```python
from build123d import *

# Parameters (mm, degrees)
PAD_DEPTH          = 5
POCKET_DEPTH       = 5.001
SKETCH002_R        = 5
POCKET001_DEPTH    = 5
SKETCH003_R        = 2.5
PAD001_DEPTH       = 15
POLARPATTERN_COUNT = 3


with BuildPart() as part:
    # Sketch → Pad (new body)
    with BuildSketch(Plane.XY):
        Polygon((0, 31.754265), (-27.5, -15.877132), (27.5, -15.877132), align=None)
    extrude(amount=PAD_DEPTH)

    # Sketch001 (on Face5 of Pad) → Pocket (cut, through all)
    with BuildSketch(Plane.XY.offset(5)):
        Polygon((-21.25, -5.051815), (-15, -15.877132), (-27.5, -15.877132), align=None)
        Polygon((27.5, -15.877132), (21.25, -5.051815), (15, -15.877132), align=None)
        Polygon((0, 31.754265), (6.25, 20.928947), (-6.25, 20.928947), align=None)
    extrude(amount=-POCKET_DEPTH, mode=Mode.SUBTRACT)

    # Sketch002 (on Face4 of Pocket) → Pocket001 (cut)
    with BuildSketch(Plane.XY.offset(5)):
        Circle(SKETCH002_R)
    extrude(amount=-POCKET001_DEPTH, mode=Mode.SUBTRACT)

    # Sketch003 → Pad001 (join, symmetric)
    with BuildSketch(Plane.YZ):
        with BuildLine():
            ThreePointArc((-16.02939, 13.038792), (-23.453338, 13.615862), (-23.218057, 6.173238))
            Line((-15.877132, 0), (-23.218057, 6.173238))
            Line((-15.877132, 5), (-15.877132, 0))
            Line((-9.877132, 5), (-15.877132, 5))
            Line((-16.02939, 13.038792), (-9.877132, 5))
        make_face()
        with Locations((-20, 10)):
            Circle(SKETCH003_R, mode=Mode.SUBTRACT)
    pad001 = extrude(amount=PAD001_DEPTH, both=True)

    # PolarPattern: Pad001 ×3 about axis
    polarpattern_axis = Axis((0, 0, 0), (0, 0, 1))
    for i in range(1, POLARPATTERN_COUNT):
        add(pad001.rotate(polarpattern_axis, i * 360 / POLARPATTERN_COUNT))


solid = part.part
```
Work out the finished part from the listing and answer in its coordinate system (mm). A direction names the side the tool comes from. Give positions to 0.01 mm unless a question says otherwise; leave off trailing zeros. Order: outer loops, then holes, each group sorted by start corner. A loop starts at its lowest first (then second) coordinate and runs counter-clockwise, first axis right, second up. Notation, with made-up numbers: M 63.25,15 L 90.25,15 A26 ccw 90.25,35 Z; hole C 57,73.25 d2. An arc over 180 degrees is marked long. Return JSON: item names as keys, results as strings.
1) For a pull along Z with two mould halves and no side action, classify faces 4 (the cylindrical face through (0, -23, 14)), 5 (the flat face through (7.69, 21.76, 7.61)), 6 (the cylindrical face through (-16.22, 9.61, 7.78)) as +Z half, -Z half, draft (parallel to the pull), parting line (faces both ways), or undercut.
Resolved:
{"face 4": "parting line", "face 5": "draft", "face 6": "undercut"}
2) Section B-B, the plane y = -20 is taken. Write down the section's boundary in (x, z), plus the area to 3 significant figures.
Resolved:
{"outline": "M -15,3.47 L 15,3.47 L 15,7.5 L -15,7.5 Z; M -15,12.5 L 15,12.5 L 15,15 L -15,15 Z", "area": "196 mm^2"}
3) Straight lines are drawn through the part: line 1 along X through (y, z) = (-1.5, 10.75); line 2 along Z through (x, y) = (-15.5, 16); line 3 along Y through (x, z) = (0, 1.95). For each, find the intervals that lie inside material, in ascending order. Write a range as [from, to].
Resolved:
{"line 1": "[-27.4, -26.71], [-21.21, -17.35], [17.35, 21.21], [26.71, 27.4]", "line 2": "[4.66, 7.94], [12.06, 14.79]", "line 3": "[-18.2, -5], [5, 20.93]"}
4) A tool of negligible diameter and unlimited length cuts with its end or side. For faces 1 (the flat face through (0.21, -13, 9.08)), 2 (the flat face through (-22.69, -4.22, 7.61)), 3 (the flat face through (-11.36, 6.32, 9.08)), from which of +Z, -Z, +X, -X, +Y, -Y can it reach the whole face along a straight path? Write none if from no direction.
Resolved:
{"face 1": "+Z, +X, -X", "face 2": "+Z, -X, -Y", "face 3": "+Z"}
5) Section C-C, the plane z = 10 is taken. Write down the section's boundary in (x, y).
Resolved:
{"outline": "M -29.15,-0.49 L -26.99,-1.74 L -11.99,24.24 L -14.15,25.49 Z; M -22.66,-4.24 L -19.37,-6.14 L -4.37,19.84 L -7.66,21.74 Z; M -15,-25 L 15,-25 L 15,-22.5 L -15,-22.5 Z; M -15,-17.5 L 15,-17.5 L 15,-13.7 L -15,-13.7 Z; M 4.37,19.84 L 19.37,-6.14 L 22.66,-4.24 L 7.66,21.74 Z; M 11.99,24.24 L 26.99,-1.74 L 29.15,-0.49 L 14.15,25.49 Z"}
6) Each of these flat-tipped pins is pushed along its axis until it touches: pin 1 (3 mm diameter, centred on x = 23, z = 6.5, fed in from -Y); pin 2 (8 mm diameter, centred on x = -7.5, z = 3.5, fed in from +Y); pin 3 (4.5 mm diameter, centred on y = -16, z = 8.5, fed in from +X). Where does it stop, or does it pass through?
Resolved:
{"pin 1": "y = -4.91", "pin 2": "y = 23.82", "pin 3": "x = 15"}
7) Section D-D, the plane y = 16.5 is taken. Give the number of separate pieces and of enclosed holes in the cut face, plus the area to 3 significant figures.
Resolved:
{"separate pieces": "1", "enclosed holes": "2", "area": "312 mm^2"}
8) Section A-A, the plane x = 0 is taken. Write down the section's boundary in (y, z).
Resolved:
{"outline": "M -23.22,6.17 L -15.88,0 L -5,0 L -5,5 L -9.88,5 L -16.03,13.04 A5 ccw long Z; M 5,0 L 20.93,0 L 20.93,5 L 5,5 Z; hole C -20,10 d5"}
